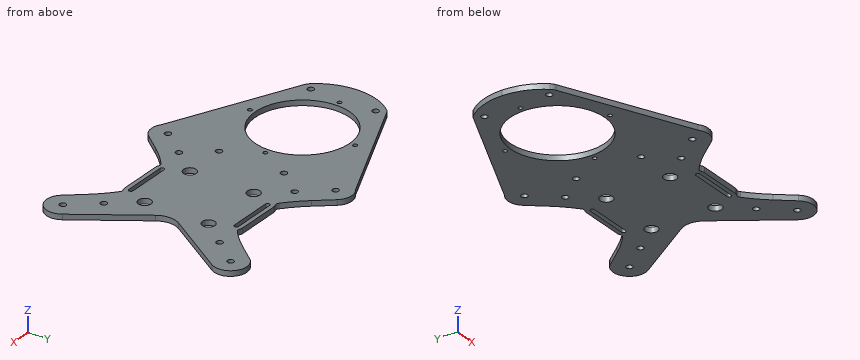
```python
from build123d import *

# Parameters (mm, degrees)
CROQUIS1_R              = 2.25
CROQUIS1_R_2            = 3
CROQUIS1_R_3            = 1.5
CROQUIS1_R_4            = 2.249997567
SALIENTE_EXTRUIR1_DEPTH = 2.5
SALIENTE_EXTRUIR3_START = -2.5
CROQUIS6_R              = 2.250000066
CROQUIS6_R_2            = 1.5
CROQUIS6_R_3            = 2.25
SALIENTE_EXTRUIR3_DEPTH = 2.5
CROQUIS5_R              = 22.5
CROQUIS5_R_2            = 1
CORTAR_EXTRUIR5_DEPTH   = 2.5


with BuildPart() as part:
    # Croquis1 → Saliente-Extruir1 (new body)
    with BuildSketch(Plane.XY):
        with BuildLine():
            Line((-29.502526327, -44.949972179), (-23.17778065, -37.243838032))
            ThreePointArc((-23.17778065, -37.243838032), (-18.839723212, -32.444384768), (-14.046056443, -28.099933953))
            ThreePointArc((-14.046056443, -28.099933953), (-12.991422185, -27.658257217), (-11.867164621, -27.866527921))
            ThreePointArc((-11.867164621, -27.866527921), (-11.203313373, -28.112469078), (-10.500314, -28.196))
            Line((-10.500314, -28.196), (10.499686, -28.196))
            ThreePointArc((10.499686, -28.196), (11.203007921, -28.112542722), (11.867164264, -27.866528101))
            ThreePointArc((11.867164264, -27.866528101), (12.991422421, -27.658256674), (14.046057406, -28.099933523))
            ThreePointArc((14.046057406, -28.099933523), (18.839775902, -32.444337151), (23.177889012, -37.243749049))
            Line((23.177889012, -37.243749049), (29.502526012, -44.949972049))
            ThreePointArc((29.502526012, -44.949972049), (40.113877497, -46.255199126), (41.931739547, -35.719556022))
            Line((41.931739547, -35.719556022), (21.72923101, -5.566101046))
            ThreePointArc((21.72923101, -5.566101046), (20.036969431, -9.5e-08), (21.729230693, 5.566100954))
            Line((21.729230693, 5.566100954), (41.931739693, 35.719555954))
            ThreePointArc((41.931739693, 35.719555954), (40.113877277, 46.255198335), (29.502526336, 44.949972165))
            Line((29.502526336, 44.949972165), (23.17778065, 37.243838007))
            ThreePointArc((23.17778065, 37.243838007), (18.839723212, 32.444384742), (14.046056443, 28.099933927))
            ThreePointArc((14.046056443, 28.099933927), (12.991421988, 27.658257139), (11.867164252, 27.866528027))
            ThreePointArc((11.867164252, 27.866528027), (11.203313175, 28.112469073), (10.500314, 28.195999974))
            Line((10.500314, 28.195999974), (-10.500314, 28.195999974))
            ThreePointArc((-10.500314, 28.195999974), (-11.203313178, 28.112469098), (-11.867164264, 27.866528075))
            ThreePointArc((-11.867164264, 27.866528075), (-12.991422421, 27.658256648), (-14.046057406, 28.099933497))
            ThreePointArc((-14.046057406, 28.099933497), (-18.839775902, 32.444337126), (-23.177889012, 37.243749023))
            Line((-23.177889012, 37.243749023), (-29.502526012, 44.949972023))
            ThreePointArc((-29.502526012, 44.949972023), (-40.146302424, 46.230987494), (-41.886340556, 35.652554517))
            ThreePointArc((-41.886340556, 35.652554517), (-41.288874902, 25.337679941), (-50.13550001, 20.000000021))
            Line((-50.13550001, 20.000000021), (-97.31807601, 20.000000021))
            ThreePointArc((-97.31807601, 20.000000021), (-99.1994919, 19.554558541), (-100.681450855, 18.312809163))
            add(Edge.make_bspline(
                [(-107.31807554, 2.1e-08), (-107.252414123, 7.059743944), (-104.975710329, 13.164639039), (-100.681450855, 18.312809163)],
                knots=[0, 0, 0, 0, 1, 1, 1, 1], degree=3))
            add(Edge.make_bspline(
                [(-107.31807554, 2.1e-08), (-107.252414123, -7.059743902), (-104.975710329, -13.164638997), (-100.681450855, -18.312809121)],
                knots=[0, 0, 0, 0, 1, 1, 1, 1], degree=3))
            ThreePointArc((-100.681450855, -18.312809121), (-99.19949186, -19.554558345), (-97.31807601, -19.9999997))
            Line((-97.31807601, -19.9999997), (-50.13550001, -19.9999997))
            ThreePointArc((-50.13550001, -19.9999997), (-41.288874902, -25.33767962), (-41.886340556, -35.652554196))
            ThreePointArc((-41.886340556, -35.652554196), (-40.146302646, -46.230987042), (-29.502526327, -44.949972179))
        make_face()
        with Locations((-25.371621, 27.641642)):
            Circle(CROQUIS1_R, mode=Mode.SUBTRACT)
        with Locations((-35.493242035, 40.033284004)):
            Circle(CROQUIS1_R, mode=Mode.SUBTRACT)
        with Locations((-35.49324201, -40.0332837)):
            Circle(CROQUIS1_R, mode=Mode.SUBTRACT)
        with Locations((15.25, -15.25)):
            Circle(CROQUIS1_R_2, mode=Mode.SUBTRACT)
        with Locations((35.493242035, -40.03328403)):
            Circle(CROQUIS1_R, mode=Mode.SUBTRACT)
        with Locations((-15.25, 15.25)):
            Circle(CROQUIS1_R_2, mode=Mode.SUBTRACT)
        with Locations((-25.371621, -27.641642)):
            Circle(CROQUIS1_R, mode=Mode.SUBTRACT)
        with Locations((-35.318076, 15.5)):
            Circle(CROQUIS1_R_3, mode=Mode.SUBTRACT)
        with Locations((25.371621, -27.641642)):
            Circle(CROQUIS1_R, mode=Mode.SUBTRACT)
        with Locations((-15.25, -15.25)):
            Circle(CROQUIS1_R_2, mode=Mode.SUBTRACT)
        with Locations((-97.318076, 15.5)):
            Circle(CROQUIS1_R_3, mode=Mode.SUBTRACT)
        with Locations((15.25, 15.25)):
            Circle(CROQUIS1_R_2, mode=Mode.SUBTRACT)
        with Locations((-35.318076, -15.5)):
            Circle(CROQUIS1_R_3, mode=Mode.SUBTRACT)
        with Locations((25.371621, 27.641642)):
            Circle(CROQUIS1_R, mode=Mode.SUBTRACT)
        with Locations((-97.318076, -15.5)):
            Circle(CROQUIS1_R_3, mode=Mode.SUBTRACT)
        with Locations((35.493241695, 40.03328329)):
            Circle(CROQUIS1_R_4, mode=Mode.SUBTRACT)
        with BuildLine():
            Line((10.499686, -24.196), (-10.500314, -24.196))
            ThreePointArc((-10.500314, -24.196), (-11.500314, -25.196), (-10.500314, -26.196))
            Line((-10.500314, -26.196), (10.499686, -26.196))
            ThreePointArc((10.499686, -26.196), (11.499686, -25.196), (10.499686, -24.196))
        make_face(mode=Mode.SUBTRACT)
        with BuildLine():
            Line((10.499686, 24.196), (-10.500314, 24.196))
            ThreePointArc((-10.500314, 24.196), (-11.500314, 25.196), (-10.500314, 26.196))
            Line((-10.500314, 26.196), (10.499686, 26.196))
            ThreePointArc((10.499686, 26.196), (11.499686, 25.196), (10.499686, 24.196))
        make_face(mode=Mode.SUBTRACT)
    extrude(amount=SALIENTE_EXTRUIR1_DEPTH)


with BuildPart() as saliente_extruir3_tool:
    # Croquis6 → Saliente-Extruir3 (new body)
    # profile 1 of 10: a face of its own
    with BuildSketch(Plane.XY.offset(2.5).offset(SALIENTE_EXTRUIR3_START)):
        with Locations((-35.493242163, 40.033284025)):
            Circle(CROQUIS6_R)
        with Locations((-35.493242163, 40.033284025)):
            Circle(CROQUIS6_R_2, mode=Mode.SUBTRACT)
    # profile 2 of 10: a face of its own
    with BuildSketch(Plane.XY.offset(2.5).offset(SALIENTE_EXTRUIR3_START)):
        with Locations((-25.371621, 27.641642)):
            Circle(CROQUIS6_R_3)
        with Locations((-25.371621, 27.641642)):
            Circle(CROQUIS6_R_2, mode=Mode.SUBTRACT)
    # profile 3 of 10: a face of its own
    with BuildSketch(Plane.XY.offset(2.5).offset(SALIENTE_EXTRUIR3_START)):
        with Locations((25.371621, 27.641642)):
            Circle(CROQUIS6_R_3)
        with Locations(Location((25.371621, 27.641642, 0), (0, 0, 180))):
            Circle(CROQUIS6_R_2, mode=Mode.SUBTRACT)
    # profile 4 of 10: a face of its own
    with BuildSketch(Plane.XY.offset(2.5).offset(SALIENTE_EXTRUIR3_START)):
        with Locations((35.493242163, 40.033284025)):
            Circle(CROQUIS6_R)
        with Locations(Location((35.493242163, 40.033284025, 0), (0, 0, 180))):
            Circle(CROQUIS6_R_2, mode=Mode.SUBTRACT)
    # profile 5 of 10: a face of its own
    with BuildSketch(Plane.XY.offset(2.5).offset(SALIENTE_EXTRUIR3_START)):
        with Locations((35.493242163, -40.033284025)):
            Circle(CROQUIS6_R)
        with Locations((35.493242163, -40.033284025)):
            Circle(CROQUIS6_R_2, mode=Mode.SUBTRACT)
    # profile 6 of 10: a face of its own
    with BuildSketch(Plane.XY.offset(2.5).offset(SALIENTE_EXTRUIR3_START)):
        with Locations((25.371621, -27.641642)):
            Circle(CROQUIS6_R_3)
        with Locations((25.371621, -27.641642)):
            Circle(CROQUIS6_R_2, mode=Mode.SUBTRACT)
    # profile 7 of 10: a face of its own
    with BuildSketch(Plane.XY.offset(2.5).offset(SALIENTE_EXTRUIR3_START)):
        with Locations((-25.371621, -27.641642)):
            Circle(CROQUIS6_R_3)
        with Locations(Location((-25.371621, -27.641642, 0), (0, 0, 180))):
            Circle(CROQUIS6_R_2, mode=Mode.SUBTRACT)
    # profile 8 of 10: a face of its own
    with BuildSketch(Plane.XY.offset(2.5).offset(SALIENTE_EXTRUIR3_START)):
        with Locations((-35.493242163, -40.033284025)):
            Circle(CROQUIS6_R)
        with Locations(Location((-35.493242163, -40.033284025, 0), (0, 0, 180))):
            Circle(CROQUIS6_R_2, mode=Mode.SUBTRACT)
    # profile 9 of 10: a face of its own
    with BuildSketch(Plane.XY.offset(2.5).offset(SALIENTE_EXTRUIR3_START)):
        with BuildLine():
            Line((-99.1994919, 19.554558541), (-40.146302424, 46.230987494))
            ThreePointArc((-40.146302424, 46.230987494), (-43.140478024, 41.291171845), (-41.886340556, 35.652554517))
            ThreePointArc((-41.886340556, 35.652554517), (-41.288875033, 25.33768001), (-50.13550001, 20.000000021))
            Line((-50.13550001, 20.000000021), (-97.31807601, 20.000000021))
            ThreePointArc((-97.31807601, 20.000000021), (-98.214581153, 19.590579436), (-99.1994919, 19.554558541))
        make_face()
    # profile 10 of 10: a face of its own
    with BuildSketch(Plane.XY.offset(2.5).offset(SALIENTE_EXTRUIR3_START)):
        with BuildLine():
            Line((-50.13550001, -20.000000021), (-97.31807601, -20.000000021))
            ThreePointArc((-97.31807601, -20.000000021), (-98.214581153, -19.590579436), (-99.1994919, -19.554558541))
            Line((-99.1994919, -19.554558541), (-40.146302424, -46.230987494))
            ThreePointArc((-40.146302424, -46.230987494), (-43.140478024, -41.291171845), (-41.886340556, -35.652554517))
            ThreePointArc((-41.886340556, -35.652554517), (-41.288875033, -25.33768001), (-50.13550001, -20.000000021))
        make_face()
    extrude(amount=SALIENTE_EXTRUIR3_DEPTH)


with BuildPart() as part_1:
    add(part.part)


with BuildPart() as part_2:
    # Saliente-Extruir3: joined with saliente_extruir3_tool
    add(part_1.part.fuse(saliente_extruir3_tool.part, tol=0.00001))

    # Croquis5 → Cortar-Extruir5 (cut)
    with BuildSketch(Plane.XY.offset(2.5)):
        with Locations((-69.81807554, 2.1e-08)):
            Circle(CROQUIS5_R)
        with Locations((-44.71807554, 2.1e-08)):
            Circle(CROQUIS5_R_2)
        with Locations((-69.81807554, -25.099999979)):
            Circle(CROQUIS5_R_2)
        with Locations((-94.91807554, 2.1e-08)):
            Circle(CROQUIS5_R_2)
        with Locations((-69.81807554, 25.100000021)):
            Circle(CROQUIS5_R_2)
    extrude(amount=-CORTAR_EXTRUIR5_DEPTH, mode=Mode.SUBTRACT)


solid = part_2.part
```
Verification items for the finished model (mm, model axes). Give positions to 0.01 mm unless a question says otherwise; leave off trailing zeros. Order: outer loops, then holes, each group sorted by start corner. A loop starts at its lowest first (then second) coordinate and runs counter-clockwise, first axis right, second up. Notation, with made-up numbers: (-20, 9.25) -> (-12, 9.25) arc R7 ccw to (-12, 18.25) -> close; hole circle Ø2 at (11.25, 11.5). An arc over 180 degrees is marked (long way). One line per item, written item: value.
(1) Sectioned sample at A-A on x = 31.5. Record the cut outline in (y, z).
Final values:
outline: (-46.68, 0) -> (-20.15, 0) -> (-20.15, 2.5) -> (-46.68, 2.5) -> close; (20.15, 0) -> (46.68, 0) -> (46.68, 2.5) -> (20.15, 2.5) -> close
(2) Sectioned sample at C-C on z = 1.95. Count the separate pieces of the cut face and the enclosed holes in it, then the cut area to 3 significant figures.
Final values:
separate pieces: 1
enclosed holes: 23
area: 7,350 mm^2
(3) Sectioned sample at B-B on y = -32.5. Record the cut outline in (x, z).
Final values:
outline: (-70.54, 0) -> (-18.9, 0) -> (-18.9, 2.5) -> (-70.54, 2.5) -> close; (18.9, 0) -> (39.77, 0) -> (39.77, 2.5) -> (18.9, 2.5) -> close
(4) Scan lines: line 1 along Y through (x, z) = (9.5, 1.55); line 2 along Y through (x, z) = (-15.25, 1.45); line 3 along Y through (x, z) = (25.5, 1.05). Record each from-to range of solid material in increasing order. Write a range as [from, to].
Final values:
line 1: [-28.2, -26.2], [-24.2, 24.2], [26.2, 28.2]
line 2: [-29.11, -18.25], [-12.25, 12.25], [18.25, 29.11]
line 3: [-40.07, -29.14], [-26.15, -11.19], [11.19, 26.15], [29.14, 40.07]
(5) Gauge pin test, flat ends, axial feed: pin 1 (0.8 mm diameter, centred on x = -3, z = 1, fed in from +Y); pin 2 (1.5 mm diameter, centred on x = -56.5, z = 2, fed in from -Y); pin 3 (8 mm diameter, centred on x = 15.25, y = 15.25, fed in from +Z); pin 4 (1 mm diameter, centred on x = -18, z = 1, fed in from +Y). Record the tip position at first contact, or that the pin passes through.
Final values:
pin 1: y = 28.2
pin 2: y = -39.18
pin 3: z = 2.5
pin 4: y = 32.11
